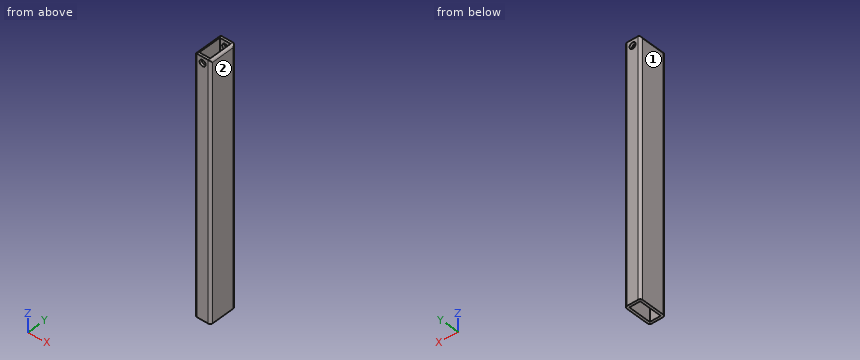
```python
from build123d import *

# Parameters (mm, degrees)
F0_W     = 33.02
F0_H     = 533.4
F1_DEPTH = 58.42
F3_T     = -5.08
F4_D     = 12.7
F5_R     = 5.07999


# Not quite as in the source:
# - a fillet or chamfer is up to 0.001 mm smaller than in the source, because OpenCascade refuses the exact size


with BuildPart() as f1:
    # F0 (on Front) → F1 (new body)
    with BuildSketch(Plane.XZ):
        with Locations((16.51, -266.7)):
            Rectangle(F0_W, F0_H)
    extrude(amount=F1_DEPTH)

    # F3
    f3_openings = [f1.faces().sort_by_distance(p)[0] for p in [
        (16.51, -29.21, 0),
        (16.51, -29.21, -533.4),
    ]]
    offset(amount=F3_T, openings=f3_openings)

    # F4 (through all)
    with Locations(Plane.XZ.offset(58.42)):
        with Locations((16.51, -12.7)):
            Hole(F4_D / 2)

    # F5 (radius 5.08 in the source; OpenCascade refuses exactly that, so slightly less here)
    f5_edges = [f1.edges().sort_by_distance(p)[0] for p in [
        (0, -58.42, -266.7),
        (33.02, -58.42, -266.7),
        (33.02, 0, -266.7),
        (0, 0, -266.7),
        (33.02, -29.21, 0),
        (0, -29.21, 0),
    ]]
    fillet(f5_edges, radius=F5_R)


solid = f1.part
```
Input: part model. Units: mm. Frame: model coordinates. Face numbers are marked on the shaded views. Coordinates: 2 decimals unless noted, no trailing zeros. Write each loop counter-clockwise with the first axis right and the second up, starting at its lowest first coordinate (ties: lowest second). Pieces come first, ordered by that corner, then holes. Notation, with made-up numbers: (42.5, 55) - (73.5, 55) arc R11 ccw to (73.5, 70) - close; hole circle Ø4 at (51.5, 79). An arc over 180 degrees is marked (long way). Put each result on its own line as item: value. Start each with the question number.
1) Ray query, L1, parallel to Y at x = 20.5, z = -282.5; L2, parallel to Z at x = 16.51, y = -2.45; L3, parallel to X at y = -31.5, z = -303. Return the intervals inside material, ascending.
2) Cut plane A-A (z = -12.7). Return the cut outline in (x, y).
3) Mould query, pull axis X, two halves, no side actions, for the marked faces 1 and 2. Classes: pulls with the +X half, pulls with the -X half, needs draft (parallel to the pull), parting line crosses it, or undercut.
4) Contact query for a flat-ended pin moving along its axis: pin 1 (10 mm diameter, centred on x = 4.5, z = -198, fed in from +Y). Output: stop coordinate, or through.
5) Cut plane C-C (x = 16.51). Return the cut outline in (y, z).
6) Cut plane D-D (z = -110.5). Return the cut outline in (x, y).
Resolved:
1. L1: y = -58.42 to -53.34, -5.08 to 0
1. L2: z = -533.4 to -19.05, -6.35 to 0
1. L3: x = 0 to 5.08, 27.94 to 33.02
2. outline: (0, -53.34) arc R5.08 ccw to (5.08, -58.42) - (10.16, -58.42) - (10.16, -53.34) - (5.08, -53.34) - (5.08, -5.08) - (10.16, -5.08) - (10.16, 0) - (5.08, 0) arc R5.08 ccw to (0, -5.08) - close; (22.86, -58.42) - (27.94, -58.42) arc R5.08 ccw to (33.02, -53.34) - (33.02, -5.08) arc R5.08 ccw to (27.94, 0) - (22.86, 0) - (22.86, -5.08) - (27.94, -5.08) - (27.94, -53.34) - (22.86, -53.34) - close
3. face 1: pulls with the -X half
3. face 2: pulls with the +X half
4. pin 1: stops at y = 0
5. outline: (-58.42, -533.4) - (-53.34, -533.4) - (-53.34, -19.05) - (-58.42, -19.05) - close; (-58.42, -6.35) - (-53.34, -6.35) - (-53.34, 0) - (-58.42, 0) - close; (-5.08, -533.4) - (0, -533.4) - (0, -19.05) - (-5.08, -19.05) - close; (-5.08, -6.35) - (0, -6.35) - (0, 0) - (-5.08, 0) - close
6. outline: (0, -53.34) arc R5.08 ccw to (5.08, -58.42) - (27.94, -58.42) arc R5.08 ccw to (33.02, -53.34) - (33.02, -5.08) arc R5.08 ccw to (27.94, 0) - (5.08, 0) arc R5.08 ccw to (0, -5.08) - close; hole (5.08, -53.34) - (27.94, -53.34) - (27.94, -5.08) - (5.08, -5.08) - close
